Autodesk Inventor part; units mm, degrees
ref_plane "YZ Plane" through (0, 0, 0) normal (1, 0, 0) x (0, 1, 0)
ref_plane "XZ Plane" through (0, 0, 0) normal (0, 1, 0) x (-1, 0, 0)
ref_plane "XY Plane" through (0, 0, 0) normal (0, 0, 1) x (1, 0, 0)
sketch "Boceto1" plane through (0, 0, 0) normal (0, 1, 0) x (-1, 0, 0)
  line L0 (-5, 22.7) -> (5, 22.7)
  line L1 (5, 22.7) -> (5, -22.7)
  line L2 (5, -22.7) -> (-5, -22.7)
  line L3 (-5, -22.7) -> (-5, 22.7)
  line L4 (-5, 22.7) -> (5, -22.7) construction
  line L5 (5, 22.7) -> (-5, -22.7) construction
  line L6 (5, 22.7) -> (-45, 22.7)
  line L7 (-45, 22.7) -> (-45, 10.2)
  line L8 (-45, 10.2) -> (5, 10.2)
  line L9 (5, 10.2) -> (5, 22.7)
  line L10 (5, -22.7) -> (-45, -22.7)
  line L11 (-45, -22.7) -> (-45, -10.2)
  line L12 (-45, -10.2) -> (5, -10.2)
  line L13 (5, -10.2) -> (5, -22.7)
  point P0 (0, 0)
  point P1 (-5, 10.2)
  point P2 (-5, -10.2)
  point P3 (-5, -22.7)
  dimension "d0" = 20.4
  dimension "d1" = 45.4
  dimension "d2" = 50
  dimension "d3" = 10
extrude "Extrusión1" add sketch "Boceto1" along normal blind 20
sketch "Boceto2" plane through (-5, 0, -22.7) normal (-1, 0, 0) x (0, 0, 1)
  circle A0 centre (22.7, 10) radius 2.7
  line L0 (0, 0) -> (45.4, 0)
  point P0 (22.7, 0)
  dimension "d6" = 5.4
  dimension "d7" = 10
extrude "Extrusión2" cut sketch "Boceto2" against normal through all
sketch "Boceto3" plane through (5, 0, 10.2) normal (1, 0, 0) x (0, 0, -1)
  point P0 (10.2, 0)
fillet "Empalme1" radius 5 2 edges at (-5, 10, -22.7) (-5, 10, 22.7)
sketch "Boceto4" plane through (0, 0, 0) normal (0, -1, 0) x (1, 0, 0)
  circle A0 centre (32.85, -16.7) radius 2.7
  circle A1 centre (32.85, 16.7) radius 2.7
  line L0 (45, -22.7) -> (0, -22.7)
  line L1 (0, 22.7) -> (45, 22.7)
  line L2 (45, 22.7) -> (45, 10.2)
  point P0 (0, 0)
  dimension "d11" = 6
  dimension "d12" = 6
  dimension "d13" = 5.4
  dimension "d19" = 12.15
extrude "Extrusión3" cut sketch "Boceto4" against normal through all
sketch "Boceto5" plane through (0, 20, 0) normal (0, 1, 0) x (1, 0, 0)
  circle A0 centre (32.85, 16.7) radius 2.7
  circle A1 centre (32.85, 16.7) radius 4.05
  circle A2 centre (32.85, -16.7) radius 2.7
  circle A3 centre (32.85, -16.7) radius 4.05
  line L0 (37.5265, 16.7) -> (35.1883, 12.65)
  line L1 (35.1883, 12.65) -> (30.5117, 12.65)
  line L2 (30.5117, 12.65) -> (28.1735, 16.7)
  line L3 (28.1735, 16.7) -> (30.5117, 20.75)
  line L4 (30.5117, 20.75) -> (35.1883, 20.75)
  line L5 (35.1883, 20.75) -> (37.5265, 16.7)
  line L6 (37.5265, -12.2178) -> (39.07, -18.5089)
  line L7 (39.07, -18.5089) -> (34.3935, -22.9911)
  line L8 (34.3935, -22.9911) -> (28.1735, -21.1822)
  line L9 (28.1735, -21.1822) -> (26.63, -14.8911)
  line L10 (26.63, -14.8911) -> (31.3065, -10.4089)
  line L11 (31.3065, -10.4089) -> (37.5265, -12.2178)
  line L12 (30.5117, -20.75) -> (28.1735, -16.7)
  line L13 (28.1735, -16.7) -> (30.5117, -12.65)
  line L14 (30.5117, -12.65) -> (35.1883, -12.65)
  line L15 (35.1883, -12.65) -> (37.5265, -16.7)
  line L16 (37.5265, -16.7) -> (35.1883, -20.75)
  line L17 (35.1883, -20.75) -> (30.5117, -20.75)
  line L18 (0, -22.7) -> (45, -22.7)
  point P0 (0, 0)
  dimension "d16" = 8.1
extrude "Extrusión4" cut sketch "Boceto5" against normal blind 4 contours A0 | A1 | A1 L5 L0 | A1 L4 L5 | L0 L1 A1 | A1 L3 L4 | L1 L2 A1 | A1 L2 L3 | A2 | A3 | A3 L15 L16 | A3 L14 L15 | L16 L17 A3 | A3 L13 L14 | L17 L12 A3 | A3 L12 L13
fillet "Empalme2" radius 5 2 edges at (45, 10, 22.7) (45, 10, -22.7)
sketch "Boceto6" plane through (5, 0, 10.2) normal (1, 0, 0) x (0, 0, -1)
  circle A0 centre (10.2, 10) radius 2.7
  circle A1 centre (10.2, 10) radius 5
  point P0 (10.2, 0)
  dimension "d21" = 10
extrude "Extrusión5" cut sketch "Boceto6" against normal blind 5 contours A0 | A1
fillet "Empalme3" radius 2 4 edges at (5, 10, -10.2) (5, 10, 10.2) (45, 10, 10.2) (45, 10, -10.2)
properties part number "Tensor"
Geometry check sheet. Reference: the model listing, model coordinates, mm. A direction names the side the tool comes from. Round coordinates to 2 decimals unless told otherwise and drop trailing zeros. Order: outer loops, then holes, each group sorted by start corner. A loop starts at its lowest first (then second) coordinate and runs counter-clockwise, first axis right, second up. Notation, with made-up numbers: M 26,-38 L 85,-38 A26 cw 85,-12 Z; hole C 81,78.25 d5. An arc over 180 degrees is marked long. Answer in a Markdown table with one row per item. Add a question column.
Item 1: Sectioned sample at D-D, the plane z = 7. Enter the section's corners in (x, y), plus the area to 3 significant figures.
Item 2: Draft check along Z on faces 4 (the face through (43.57, 10.14, -21.2)), 5 (the face through (34, 16, 14)), 6 (the face through (14.8, 20, 10.4)). Enter one of: released by +Z, released by -Z, zero draft, split by the parting line, or undercut.
Item 3: Sectioned sample at A-A, the plane y = 10. Enter the section's corners in (x, z), plus the area to 3 significant figures.
Item 4: Sectioned sample at B-B, the plane z = 0. Enter the section's corners in (x, y), plus the area to 3 significant figures.
Item 5: Depth check by flat-ended pin: pin 1 Ø4 at (y, z) = (5.5, -6) entering from +X; pin 2 Ø8 at (y, z) = (10, 0) entering from +X; pin 3 Ø2.5 at (x, z) = (34.5, 18) entering from +Y. Enter the tip coordinate at first touch or a pass-through.
Item 6: Material ranges on L1, parallel to Z at x = 32.85, y = 8.75; L2, parallel to Z at x = 11, y = 4.5; L3, parallel to Y at x = -2.6, z = 0, recorded low to high. Write a range as [from, to].
Item 7: Sectioned sample at C-C, the plane x = 23. Enter the section's corners in (y, z), plus the area to 3 significant figures.
Item 8: Set-up check for faces 1 (the face through (5.6, 10.14, -9.63)), 2 (the face through (33, 18, -20.75)), 3 (the face through (0, 7.8, -2.2)): record each of +Z, -Z, +X, -X, +Y, -Y from which the full face is reachable in a straight line by a thin tool's end or side.
Filled in:
| question | item | result |
|---|---|---|
| 1 | outline | M -5,0 L 5,0 L 5,20 L -5,20 Z |
| 1 | area | 200 mm² |
| 2 | face 4 | released by -Z |
| 2 | face 5 | undercut |
| 2 | face 6 | zero draft |
| 3 | outline | M -5,-17.7 A5 ccw 0,-22.7 L 40,-22.7 A5 ccw 45,-17.7 L 45,-12.2 A2 ccw 43,-10.2 L 7,-10.2 A2 cw 5,-8.2 L 5,-5 L 0,-5 L 0,-2.7 L -5,-2.7 Z; M -5,2.7 L 0,2.7 L 0,5 L 5,5 L 5,8.2 A2 cw 7,10.2 L 43,10.2 A2 ccw 45,12.2 L 45,17.7 A5 ccw 40,22.7 L 0,22.7 A5 ccw -5,17.7 Z; hole C 32.85,-16.7 d5.4; hole C 32.85,16.7 d5.4 |
| 3 | area | 1,310 mm² |
| 4 | outline | M -5,0 L 5,0 L 5,5 L 0,5 L 0,7.3 L -5,7.3 Z; M -5,12.7 L 0,12.7 L 0,15 L 5,15 L 5,20 L -5,20 Z |
| 4 | area | 123 mm² |
| 5 | pin 1 | stops at x = 5 |
| 5 | pin 2 | stops at x = 0 |
| 5 | pin 3 | stops at y = 16 |
| 6 | L1 | z = [-22.7, -19.4], [-14, -10.2], [10.2, 14], [19.4, 22.7] |
| 6 | L2 | z = [-22.7, -10.2], [10.2, 22.7] |
| 6 | L3 | y = [0, 7.3], [12.7, 20] |
| 7 | outline | M 0,-22.7 L 20,-22.7 L 20,-10.2 L 0,-10.2 Z; M 0,10.2 L 20,10.2 L 20,22.7 L 0,22.7 Z |
| 7 | area | 500 mm² |
| 8 | face 1 | +X, +Y, -Y |
| 8 | face 2 | +Y |
| 8 | face 3 | +X |
